from build123d import *

# Parameters (mm, degrees)
SKETCH2_W           = 85
SKETCH2_H           = 78
BOSS_EXTRUDE2_DEPTH = 3
SKETCH5_R           = 2.5
CUT_EXTRUDE1_DEPTH  = 3
FILLET1_R           = 5
FILLET2_R           = 5
FILLET3_R           = 5
FILLET4_R           = 5
SKETCH12_W          = 10
SKETCH12_H          = 2.5
BOSS_EXTRUDE3_DEPTH = 3
SKETCH14_W          = 10
SKETCH14_H          = 2
BOSS_EXTRUDE4_DEPTH = 1.5
FILLET10_R          = 0.5
FILLET11_START      = 47
FILLET11_DEPTH      = 11


with BuildPart() as part:
    # Sketch2 → Boss-Extrude2 (new body)
    with BuildSketch(Plane.XY):
        with Locations((32.5, -1)):
            Rectangle(SKETCH2_W, SKETCH2_H)
    extrude(amount=BOSS_EXTRUDE2_DEPTH)

    # Sketch5 → Cut-Extrude1 (cut)
    with BuildSketch(Plane.XY):
        with Locations((-6, -36)):
            Circle(SKETCH5_R)
        with Locations((71, -36)):
            Circle(SKETCH5_R)
    extrude(amount=CUT_EXTRUDE1_DEPTH, mode=Mode.SUBTRACT)

    # Fillet1
    fillet1_edges = [part.edges().sort_by_distance(p)[0] for p in [
        (75, -40, 1.5),
    ]]
    fillet(fillet1_edges, radius=FILLET1_R)

    # Fillet2
    fillet2_edges = [part.edges().sort_by_distance(p)[0] for p in [
        (75, 38, 1.5),
    ]]
    fillet(fillet2_edges, radius=FILLET2_R)

    # Fillet3
    fillet3_edges = [part.edges().sort_by_distance(p)[0] for p in [
        (-10, 38, 1.5),
    ]]
    fillet(fillet3_edges, radius=FILLET3_R)

    # Fillet4
    fillet4_edges = [part.edges().sort_by_distance(p)[0] for p in [
        (-10, -40, 1.5),
    ]]
    fillet(fillet4_edges, radius=FILLET4_R)

    # Sketch12 → Boss-Extrude3 (add)
    with BuildSketch(Plane.XY):
        with Locations((52.5, 34.75)):
            Rectangle(SKETCH12_W, SKETCH12_H)
    extrude(amount=-BOSS_EXTRUDE3_DEPTH)

    # Sketch14 → Boss-Extrude4 (add)
    with BuildSketch(Plane(origin=(0, 36, 0), x_dir=(1, 0, 0), z_dir=(0, 1, 0))):
        with Locations((52.5, 2)):
            Rectangle(SKETCH14_W, SKETCH14_H)
    extrude(amount=BOSS_EXTRUDE4_DEPTH)

    # Fillet10
    fillet10_edges = [part.edges().sort_by_distance(p)[0] for p in [
        (57.5, 35.5, -3),
        (52.5, 33.5, -3),
        (57.5, 33.5, -1.5),
        (47.5, 35.5, -3),
        (47.5, 33.5, -1.5),
        (57.5, 34.75, 0),
        (52.5, 36, 0),
        (47.5, 34.75, 0),
        (52.5, 33.5, 0),
        (57.5, 36, -0.5),
        (47.5, 36, -0.5),
        (47.5, 36.75, -1),
        (57.5, 36.75, -1),
        (47.5, 37.5, -2),
        (57.5, 37.5, -2),
    ]]
    fillet(fillet10_edges, radius=FILLET10_R)

    # Fillet11: read off the stored shape, not the designer's step
    # Fillet11 outline → Fillet11 (cut)
    with BuildSketch(Plane.YZ.offset(FILLET11_START)):
        with BuildLine():
            add(Edge.make_bspline(
                [(34.5, -3), (37.5, -3), (37.5, -1.7)],
                knots=[0, 0, 0, 1, 1, 1], degree=2, weights=[1, 0.707106781, 1]))
            Line((34.5, -3), (37.5, -3))
            Line((37.5, -3), (37.5, -1.7))
        make_face()
    extrude(amount=FILLET11_DEPTH, mode=Mode.SUBTRACT)


solid = part.part
Work out the finished part from the listing and answer in its coordinate system (mm). A direction names the side the tool comes from. Give positions to 0.01 mm unless a question says otherwise; leave off trailing zeros. Loops run counter-clockwise (first coordinate to the right, second up) from the corner with the lowest first, then second, coordinate; pieces in that order, holes last. Notation, with made-up numbers: (-29, 69.5) -> (12, 69.5) arc R17 ccw to (12, 94.5) -> close; hole circle Ø1 at (18.25, 5.25). An arc over 180 degrees is marked (long way). Use a Markdown table: item, result. Add a question column.
1. Determine the mould class of faces 1 (the cylindrical face through (74, 36, 2)), 2 (the cylindrical face through (-4.66, -33.89, 1.48)), 3 (the cylindrical face through (69.16, -34.31, 1.48)), 4 (the cylindrical face through (-9, -38, 2)) for opening direction Y: released by +Y, released by -Y, zero draft, split by the parting line, or undercut.
2. Flat-ended cylindrical pins translate along their axes: pin 1 Ø0.6 at (x, z) = (52, -1.5) entering from -Y; pin 2 Ø23.5 at (x, y) = (43, 4) entering from -Z; pin 3 Ø1.6 at (y, z) = (35.5, -2) entering from -X; pin 4 Ø4.5 at (x, y) = (71, -36) entering from +Z. Find the tip coordinate at first contact, or state that the pin passes through.
3. Section A-A on x = -6 is taken. Determine the outline of the cut face in (y, z).
4. Section B-B on y = -36 is taken. Determine the outline of the cut face in (x, z), and give its area (3 significant figures).
5. For faces 5 (the flat face through (52, 33.5, -1)), 6 (the cylindrical face through (-8, 37, 2)), 7 (the flat face through (47.5, 35, -2)), 8 (the flat face through (57.5, 35, -2)), determine the directions among +Z, -Z, +X, -X, +Y, -Y from which every point of the face is accessible in a straight line to the end or side of a thin tool.
6. Find the intervals of material crossed by probe 1 along Z at (x, y) = (70, -12.5); probe 2 along Y at (x, z) = (-5.5, 1); probe 3 along Y at (x, z) = (71, 1.3), in increasing order.
7. Section C-C on x = 23 is taken. Determine the outline of the cut face in (y, z).
8. Section D-D on y = -25 is taken. Determine the outline of the cut face in (x, z).
Results below:
| question | item | result |
|---|---|---|
| 1 | face 1 | released by +Y |
| 1 | face 2 | undercut |
| 1 | face 3 | undercut |
| 1 | face 4 | released by -Y |
| 2 | pin 1 | stops at y = 33.5 |
| 2 | pin 2 | stops at z = 0 |
| 2 | pin 3 | stops at x = 47.5 |
| 2 | pin 4 | passes through |
| 3 | outline | (-39.9, 0) -> (-38.5, 0) -> (-38.5, 3) -> (-39.9, 3) -> close; (-33.5, 0) -> (37.9, 0) -> (37.9, 3) -> (-33.5, 3) -> close |
| 4 | outline | (-9.9, 0) -> (-8.5, 0) -> (-8.5, 3) -> (-9.9, 3) -> close; (-3.5, 0) -> (68.5, 0) -> (68.5, 3) -> (-3.5, 3) -> close; (73.5, 0) -> (74.9, 0) -> (74.9, 3) -> (73.5, 3) -> close |
| 4 | area | 224 mm^2 |
| 5 | face 5 | -Z, +X, -X, -Y |
| 5 | face 6 | +Z, -Z, -X, +Y |
| 5 | face 7 | -Z, -X, +Y, -Y |
| 5 | face 8 | -Z, +X, +Y, -Y |
| 6 | probe 1 | z = 0 to 3 |
| 6 | probe 2 | y = -39.97 to -38.45, -33.55 to 37.97 |
| 6 | probe 3 | y = -39.9 to -38.5, -33.5 to 37.9 |
| 7 | outline | (-40, 0) -> (38, 0) -> (38, 3) -> (-40, 3) -> close |
| 8 | outline | (-10, 0) -> (75, 0) -> (75, 3) -> (-10, 3) -> close |
